For this review, take the finished solid that the model builds, in its own axes (mm). Face numbers are marked on the shaded views. A direction names the side the tool comes from. Coordinates: 2 decimals unless noted, no trailing zeros. Write each loop counter-clockwise with the first axis right and the second up, starting at its lowest first coordinate (ties: lowest second). Pieces come first, ordered by that corner, then holes. Notation, with made-up numbers: (86, 33.25) - (98, 33.25) arc R7 ccw to (98, 39.25) - close; hole circle Ø11 at (64, 89). An arc over 180 degrees is marked (long way). Use one line per item in the form item = value. Start each with the question number.
1) For L1, parallel to Y at x = 81.2, z = -5; L2, parallel to X at y = -126, z = -8.5; L3, parallel to Z at x = 65.75, y = -112, list the stretches that pass through material, from the lowest coordinate up. Write a range as from..to.
2) Mouldability with a two-part tool opening along Y and no side actions: class the marked faces 1, 2 and 3 as pulls with the +Y half, pulls with the -Y half, needs draft (parallel to the pull), parting line crosses it, or undercut.
3) Tool access review of the marked faces 4, 5, 6 and 7: name each direction out of +Z, -Z, +X, -X, +Y, -Y from which nothing blocks a thin tool from reaching the whole face with its end or side.
4) Insertion check: P1, Ø2, axis at x = 74, y = -99, coming from the -Z side; P2, Ø9, axis at x = 73, y = -88, coming from the -Z side; P3, Ø7.5, axis at y = -88.5, z = 2.5, coming from the +X side; P4, Ø3, axis at x = 72, y = -126, coming from the +Z side. Each pin has a flat end and moves straight along its axis. Give the tip position at first contact, or say it passes through.
5) We need section B-B (y = -107). Give the boundary of the cut face in (x, z), plus the area to 3 significant figures.
6) We need section A-A (z = -5). Give the boundary of the cut face in (x, y), plus the area to 3 significant figures.
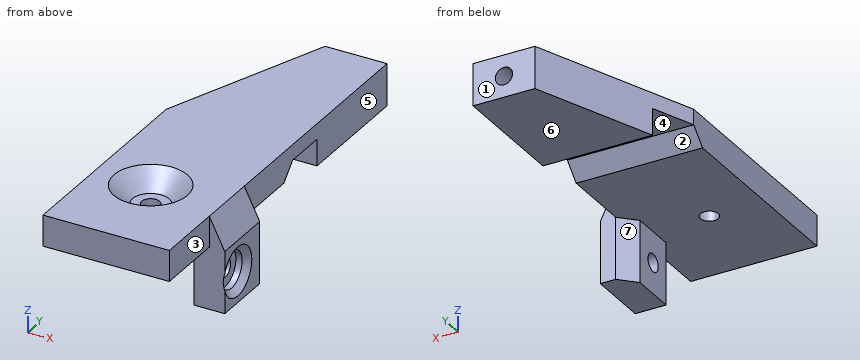
Autodesk Inventor part; units mm, degrees
ref_plane "YZ Plane" through (0, 0, 0) normal (1, 0, 0) x (0, 1, 0)
ref_plane "XZ Plane" through (0, 0, 0) normal (0, 1, 0) x (-1, 0, 0)
ref_plane "XY Plane" through (0, 0, 0) normal (0, 0, 1) x (1, 0, 0)
sketch "Esboço1" plane through (0, 0, 0) normal (0, 0, 1) x (1, 0, 0)
  line L0 (80.2817, -126.5075) -> (80.2817, -137.9075)
  line L1 (80.2817, -137.9075) -> (59.6627, -137.9075)
  line L2 (77.7817, -126.5075) -> (80.2817, -126.5075)
  line L3 (77.7817, -119.0075) -> (77.7817, -126.5075)
  line L4 (59.6627, -137.9075) -> (59.6627, -102.6075)
  line L5 (80.2817, -116.5075) -> (77.7817, -119.0075)
  line L6 (59.6627, -102.6075) -> (80.2817, -102.6075)
  line L7 (80.2817, -105.1075) -> (80.2817, -116.5075)
  line L8 (80.2817, -102.6075) -> (80.2817, -105.1075)
  line L9 (77.7817, -122.7575) -> (59.6627, -122.7575)
  circle A0 centre (68.7222, -122.7575) radius 1.45
  point P0 (0, 0)
  dimension "d65" = 2.9
extrude "Extrusão1" add sketch "Esboço1" along normal blind 5 contours L0 L1 L4 L9 A0 L3 L2 | L9 A0 L4 L6 L8 L7 L5 L3
sketch "Esboço2" plane through (0, 0, 5) normal (0, 0, 1) x (1, 0, 0)
  line L0 (69.9722, -137.7075) -> (80.6667, -137.7075)
  line L1 (80.6667, -137.7075) -> (80.6667, -138.3178)
  line L2 (80.6667, -138.3178) -> (69.9722, -138.3178)
  line L3 (69.9722, -137.7075) -> (59.8627, -137.7075)
  line L4 (59.358, -137.7075) -> (59.358, -138.3178)
  line L5 (59.358, -138.3178) -> (69.9722, -138.3178)
  line L6 (69.9722, -102.8075) -> (80.6667, -102.8075)
  line L7 (80.6667, -102.8075) -> (80.6667, -102.3974)
  line L8 (80.6667, -102.3974) -> (69.9722, -102.3974)
  line L9 (69.9722, -102.8075) -> (59.8627, -102.8075)
  line L10 (59.358, -102.8075) -> (59.358, -102.3974)
  line L11 (59.358, -102.3974) -> (69.9722, -102.3974)
  line L12 (59.358, -102.6075) -> (59.358, -138.3178)
  line L13 (59.358, -138.3178) -> (59.8627, -138.3178)
  line L14 (59.8627, -137.7075) -> (59.8627, -102.8075)
  point P0 (0, 0)
extrude "Extrusão2" cut sketch "Esboço2" against normal through all
sketch "Esboço3" plane through (80.2817, -116.5075, 5) normal (1, 0, 0) x (0, 0, -1)
  line L0 (5, 0) -> (5, 13.7)
  line L1 (5, 13.7) -> (2.5, 13.7)
  line L2 (5, 13.7) -> (0, 13.7)
  line L3 (5, 13.7) -> (5, 11.2)
  line L4 (2.5, 13.7) -> (5, 11.2)
  point P0 (5, 116.5075)
  dimension "d15" = 2.5
  dimension "d16" = 2.5
extrude "Extrusão3" cut sketch "Esboço3" against normal through all
sketch "Esboço4" plane through (0, 0, 0) normal (0, 0, -1) x (-1, 0, 0)
  line L0 (-77.7817, -119.0075) -> (-80.2817, -116.5075)
  line L1 (-77.7817, -126.5075) -> (-77.7817, -119.0075)
  line L2 (-80.2817, -116.5075) -> (-77.7817, -119.0075)
  line L3 (-77.7817, -119.0075) -> (-77.7817, -126.5075)
  line L4 (-77.7817, -126.5075) -> (-80.2817, -126.5075)
  line L5 (-80.2817, -126.5075) -> (-80.2817, -116.5075)
  point P0 (0, 0)
extrude "Extrusão4" add sketch "Esboço4" along normal blind 10
sketch "Esboço5" plane through (0, 0, -10) normal (0, 0, -1) x (-1, 0, 0)
  line L0 (-77.7817, -119.0075) -> (-80.2817, -116.5075)
  line L1 (-80.2817, -116.5075) -> (-80.2817, -116.6075)
  line L2 (-80.2817, -116.6075) -> (-77.7817, -119.1075)
  line L3 (-80.2817, -116.5075) -> (-80.2817, -126.5075)
  line L4 (-80.2817, -116.5075) -> (-80.2817, -116.1602)
  line L5 (-80.2817, -116.5075) -> (-80.2817, -105.3075)
  line L6 (-80.2817, -116.1602) -> (-77.7817, -116.1602)
  line L7 (-77.7817, -116.1602) -> (-77.7817, -119.1075)
  line L8 (-80.2817, -126.5075) -> (-80.2817, -126.4075)
  line L9 (-80.2817, -126.4075) -> (-77.6383, -126.4075)
  line L10 (-77.6383, -126.4075) -> (-77.6383, -126.5963)
  line L11 (-77.6383, -126.5963) -> (-80.2817, -126.5963)
  line L12 (-80.2817, -126.5963) -> (-80.2817, -126.4075)
  point P0 (0, 0)
  dimension "d26" = 0.1
extrude "Extrusão5" cut sketch "Esboço5" against normal blind 10 contours L0 L4 L6 L7 | L9 L10 L11 L12 L3
sketch "Esboço6" plane through (0, 0, 5) normal (0, 0, 1) x (1, 0, 0)
  line L0 (80.2817, -126.5075) -> (77.7817, -126.5075)
  line L1 (80.2817, -126.5075) -> (77.7817, -126.5075)
  line L2 (77.7817, -119.0075) -> (80.2817, -116.5075)
  line L3 (77.7817, -126.5075) -> (77.7817, -119.0075)
  line L4 (77.7817, -119.0075) -> (80.2817, -116.5075)
  line L5 (80.2817, -116.5075) -> (80.2817, -126.5075)
  point P0 (0, 0)
extrude "Extrusão6" add sketch "Esboço6" against normal blind 5
sketch "Esboço7" plane through (80.2817, -137.7075, 5) normal (1, 0, 0) x (0, 0, -1)
  line L0 (5, 21.2) -> (15, 21.2)
  line L1 (15, 21.2) -> (15, 18.7)
  line L2 (15, 21.2) -> (15, 11.3)
  line L3 (5, 18.7) -> (5, 21.2)
  line L4 (15, 18.7) -> (5, 18.7)
  line L5 (5, 18.7) -> (5, 21.2)
  line L6 (5, 21.2) -> (15, 21.2)
  line L7 (15, 11.3) -> (5, 11.3)
  line L8 (5, 11.3) -> (15, 18.7)
  circle A0 centre (10, 15) radius 1.45
  point P0 (5, 137.7075)
  dimension "d31" = 2.5
  dimension "d32" = 2.9
extrude "Extrusão7" cut sketch "Esboço7" against normal blind 5 contours A0 L8 | L8 A0
sketch "Esboço8" plane through (0, 0, 5) normal (0, 0, 1) x (1, 0, 0)
  line L0 (80.2817, -137.7075) -> (80.2817, -102.8075)
  line L1 (80.2817, -102.8075) -> (80.2817, -95.9075)
  line L2 (80.2817, -95.9075) -> (50.2817, -95.9075)
  line L3 (50.2817, -95.9075) -> (50.2817, -102.8075)
  line L4 (80.2817, -102.8075) -> (59.8627, -102.8075)
  line L5 (50.2817, -102.8075) -> (80.2817, -102.8075)
  point P0 (0, 0)
  dimension "d35" = 6.9
  dimension "d36" = 30
extrude "Extrusão8" add sketch "Esboço8" against normal blind 2.5
sketch "Esboço10" plane through (50.2817, -95.9075, 5) normal (0, 1, 0) x (1, 0, 0)
  line L0 (30, 0) -> (30, 2.5)
  line L1 (30, 5) -> (30, 2.5)
  line L2 (30, 0) -> (30, 2.5)
  line L3 (30, 2.5) -> (30, 6.8)
  line L4 (30, 6.8) -> (0, 6.8)
  line L5 (0, 0) -> (0, 2.5)
  line L6 (0, 6.8) -> (0, 0)
  line L7 (0, 0) -> (30, 0)
  point P0 (-50.2817, 5)
  dimension "d39" = 4.3
extrude "Extrusão9" add sketch "Esboço10" along normal blind 2.5
sketch "Esboço11" plane through (50.2817, -93.4075, 5) normal (0, 1, 0) x (1, 0, 0)
  line L0 (30, 2.5) -> (30, 6.8)
  line L1 (30, 5) -> (30, 2.5)
  line L2 (30, 6.8) -> (30, 2.5)
  line L3 (0, 0) -> (0, 2.5)
  line L4 (30, 2.5) -> (0, 2.5)
  line L5 (0, 6.8) -> (0, 2.5)
  line L6 (0, 2.5) -> (0, 6.8)
  line L7 (0, 6.8) -> (30, 6.8)
  line L8 (0, 2.5) -> (30, 2.5)
  line L9 (30, 2.5) -> (30, 0)
  line L10 (30, 0) -> (0, 0)
  line L11 (0, 0) -> (0, 2.5)
  point P0 (-50.2817, 5)
  dimension "d42" = 4.3
extrude "Extrusão10" add sketch "Esboço11" along normal blind 12.3
sketch "Esboço12" plane through (80.2817, -95.9075, -1.8) normal (0, 0, -1) x (-1, 0, 0)
  line L0 (0, 14.8) -> (30, 14.8)
  line L1 (0, 14.8) -> (30, 14.8)
  line L2 (30, 14.8) -> (30, 19.8)
  line L3 (30, 19.8) -> (0, 19.8)
  line L4 (0, 19.8) -> (0, 14.8)
  point P0 (80.2817, 95.9075)
  dimension "d45" = 5
extrude "Extrusão11" add sketch "Esboço12" against normal blind 6.8
sketch "Esboço14" plane through (80.2817, -137.7075, 5) normal (1, 0, 0) x (0, 0, -1)
  line L0 (5, 18.7) -> (5, 21.2)
  line L1 (15, 21.2) -> (15, 11.3)
  line L2 (5, 21.2) -> (15, 21.2)
  line L3 (15, 21.2) -> (15, 11.3)
  line L4 (15, 11.3) -> (5, 11.3)
  line L5 (5, 11.3) -> (5, 21.2)
  circle A0 centre (10, 15) radius 1.45
  circle A1 centre (10, 15) radius 1.45
  point P0 (5, 137.7075)
extrude "Extrusão13" add sketch "Esboço14" along normal blind 2.5
sketch "Esboço15" plane through (77.7817, -126.4075, -10) normal (0, -1, 0) x (1, 0, 0)
  line L0 (5, 10) -> (5, 0)
  line L1 (2.5, 15) -> (2.5, 10)
  line L2 (5, 10) -> (2.5, 10)
  line L3 (2.5, 10) -> (2.5, 15)
  line L4 (2.5, 15) -> (5, 10)
  point P0 (-77.7817, 10)
extrude "Extrusão14" add sketch "Esboço15" against normal blind 9.9
sketch "Esboço16" plane through (50.2817, -76.1075, -1.8) normal (0, 1, 0) x (1, 0, 0)
  line L0 (30, 0) -> (0, 0)
  line L1 (15, 0) -> (15, -6.8)
  line L2 (9.581, -6.8) -> (30, -6.8)
  line L3 (15, -3.4) -> (30, -3.4)
  line L4 (30, -3.4) -> (25, -3.4)
  circle A0 centre (25, -3.4) radius 1.4
  point P0 (-50.2817, -1.8)
  dimension "d92" = 5
  dimension "d99" = 2.8
extrude "Extrusão15" cut sketch "Esboço16" against normal blind 10
sketch "Esboço18" plane through (0, 0, 5) normal (0, 0, 1) x (1, 0, 0)
  line L0 (80.2817, -116.5075) -> (80.2817, -76.1075)
  line L1 (80.2817, -76.1075) -> (70.2817, -76.1075)
  line L2 (50.2817, -76.1075) -> (80.2817, -76.1075)
  line L3 (80.2817, -102.8075) -> (59.8627, -102.8075)
  line L4 (70.2817, -76.1075) -> (59.8627, -102.8075)
  line L5 (59.8627, -102.8075) -> (80.2817, -102.8075)
  line L6 (80.2817, -102.8075) -> (80.2817, -76.1075)
  line L7 (70.2817, -76.1075) -> (50.2817, -76.1075)
  line L8 (50.2817, -76.1075) -> (50.2817, -102.8075)
  line L9 (50.2817, -102.8075) -> (59.8627, -102.8075)
  line L10 (50.2817, -102.8075) -> (50.2817, -76.1075)
  point P0 (0, 0)
  dimension "d96" = 10
extrude "Extrusão16" cut sketch "Esboço18" against normal through all contours L9 L8 L2 L4
sketch "Esboço19" plane through (0, 0, 5) normal (0, 0, 1) x (1, 0, 0)
  circle A0 centre (68.7222, -122.7575) radius 1.45
  circle A1 centre (68.7222, -122.7575) radius 1.45
  circle A2 centre (68.7222, -122.7575) radius 2.95
  point P0 (0, 0)
  dimension "d100" = 5.9
extrude "Extrusão17" cut sketch "Esboço19" against normal blind 3
chamfer "Chanfro9" distance 3 angle 45 1 edges at (65.7722, -122.7575, 5)
sketch "Esboço20" plane through (82.7817, -137.7075, 5) normal (1, 0, 0) x (0, 0, -1)
  circle A0 centre (10, 15) radius 1.45
  circle A1 centre (10, 15) radius 1.45
  circle A2 centre (10, 15) radius 2.95
  point P0 (5, 137.7075)
  dimension "d106" = 5.9
extrude "Extrusão18" cut sketch "Esboço20" against normal blind 2
chamfer "Chanfro10" distance 1 angle 45 1 edges at (82.7817, -122.7075, -2.05)
properties part number "suporte_esquerdo"
Determined:
q1.L1 = -126.41..-125.66, -119.76..-116.51
q1.L2 = 77.78..82.78
q1.L3 = 0..5
q2.face_1 = pulls with the +Y half
q2.face_2 = undercut
q2.face_3 = needs draft
q3.face_4 = -Z, +X, -X
q3.face_5 = +Z, -Z, +X, +Y
q3.face_6 = -Z, +X, -X, +Y
q3.face_7 = -Z, -X
q4.P1 = 2.5
q4.P2 = -1.8
q4.P3 = 80.28
q4.P4 = 5
q5.outline = (59.86, 0) - (80.28, 0) - (80.28, 5) - (59.86, 5) - close
q5.area = 102 mm²
q6.outline = (77.78, -126.41) - (82.53, -126.41) - (81.78, -125.66) - (80.78, -125.66) - (80.78, -124.16) - (77.78, -124.16) - close; (77.78, -121.26) - (80.78, -121.26) - (80.78, -119.76) - (81.78, -119.76) - (82.78, -118.76) - (82.78, -116.51) - (80.28, -116.51) - (77.78, -119.01) - close
q6.area = 24.9 mm²
